```python
from build123d import *


with BuildPart() as part:
    # Sketch1 → Revolve3 (revolve)
    with BuildSketch(Plane(origin=(0, 0, 0), x_dir=(1, 0, 0), z_dir=(0, 1, 0))):
        with BuildLine():
            Line((-1.932900288, -25.23044077), (-49.062545314, -15.212725471))
            ThreePointArc((-49.062545314, -15.212725471), (-50.375512304, -15.004771929), (-51.703023788, -14.9352))
            Line((-51.703023788, -14.9352), (-60.325, -14.9352))
            ThreePointArc((-60.325, -14.9352), (-62.57006403, -15.86513597), (-63.5, -18.1102))
            Line((-63.5, -18.1102), (-63.5, -25.4))
            Line((-63.5, -25.4), (-76.2, -25.4))
            Line((-76.2, -25.4), (-76.2, -9.525))
            Line((-76.2, -9.525), (-63.5, -9.525))
            Line((-63.5, -9.525), (-63.5, -10.16))
            Line((-63.5, -10.16), (-51.201130044, -10.16))
            ThreePointArc((-51.201130044, -10.16), (-49.87361856, -10.229571929), (-48.56065157, -10.437525471))
            Line((-48.56065157, -10.437525471), (-1.267499712, -20.48999522))
            ThreePointArc((-1.267499712, -20.48999522), (-0.356611032, -21.048188521), (0, -22.055227011))
            Line((0, -22.055227011), (0, -23.66520898))
            ThreePointArc((0, -23.66520898), (-0.59316151, -24.908797947), (-1.932900288, -25.23044077))
        make_face()
    revolve(axis=Axis((88.99, 0, 0), (-1, 0, 0)))


solid = part.part
```
Could you check a few things on this model? Use its own coordinates, in mm. A direction names the side the tool comes from. Give positions to 0.01 mm unless a question says otherwise; leave off trailing zeros. Loops run counter-clockwise (first coordinate to the right, second up) from the corner with the lowest first, then second, coordinate; pieces in that order, holes last. Notation, with made-up numbers: (-17, -19) - (35, -19) arc R18 cw to (35, 12) - close; hole circle Ø3 at (72, 83). An arc over 180 degrees is marked (long way). Use one line per item in the form item = value.
1. I need wall thicknesses on probe 1 along Y at (x, z) = (-68, 0) (3 decimals); probe 2 along Y at (x, z) = (-60, 0); probe 3 along Z at (x, y) = (-54, -9). Which ranges of each line are inside material? Lowest first, please.
Response values:
probe_1 = -25.4 to -9.525, 9.525 to 25.4
probe_2 = -14.94 to -10.16, 10.16 to 14.94
probe_3 = -11.92 to -4.71, 4.71 to 11.92
2. On a 3-axis mill with a long thin cutter (end or side, diameter ignored), from which of +Z, -Z, +X, -X, +Y, -Y can I reach the whole of each face in a straight line? I mean faces 1 (the face through (-57.264, 10.074, -1.323)), 2 (the face through (0, -16, -16)), 3 (the face through (-63.5, 17.3, 6)). Say none if no direction works.
Response values:
face_1 = +X
face_2 = +Z, -Z, +X, +Y, -Y
face_3 = none
3. Thinking about a two-plate mould opening in X: for faces 4 (the face through (-76.2, 0, 11)), 5 (the face through (-69.761, -5.796, -7.559)), 6 (the face through (-31.064, 18.876, -2.478)), which applies, released by +X, released by -X, zero draft, split by the parting line, or undercut?
Response values:
face_4 = released by -X
face_5 = zero draft
face_6 = undercut
4. I want a section at C-C (x = -31.5). Please give me the cut outline in (y, z).
Response values:
outline = circle Ø37.89 at (0, 0); hole circle Ø28.13 at (0, 0)
5. I'm going to push flat-ended pins straight in: pin 1 Ø3 at (x, y) = (-20.5, 10.5) entering from -Z; pin 2 Ø6 at (x, z) = (-50.5, 16.5) entering from -Y; pin 3 Ø6 at (x, y) = (-29.5, -8) entering from -Z. Where does each tip first touch, or does it pass through?
Response values:
pin_1 = -19.37
pin_2 = -6.57
pin_3 = -18.94
6. I want a section at D-D (x = -5.5). Please give me the cut outline in (y, z), and give its area (3 significant figures).
Response values:
outline = circle Ø48.94 at (0, 0); hole circle Ø39.18 at (0, 0)
area = 676 mm²
